CAD build for the part. Positions are in the model's coordinates, mm. A direction names the side the tool comes from. Give positions to 0.01 mm unless a question says otherwise; leave off trailing zeros. Order: outer loops, then holes, each group sorted by start corner. A loop starts at its lowest first (then second) coordinate and runs counter-clockwise, first axis right, second up. Notation, with made-up numbers: (24, 87.25) -> (83, 87.25) arc R25 cw to (83, 118.25) -> close; hole circle Ø9 at (1, 35). An arc over 180 degrees is marked (long way). Use one line per item in the form item = value. Start each with the question number.
1) Tool access for faces 4 (the face through (-4.705, -8, 7)), 5 (the face through (-22.305, 10, 7)), 6 (the face through (-1.188, -8, 7)): list every direction of +Z, -Z, +X, -X, +Y, -Y with a clear straight run to the whole face (end or side of a thin tool).
2) Cut at A-A, the plane x = -3.75. Give the cut face in (y, z).
3) Drop flat-ended pins along their axis: P1, Ø3, axis at y = -5, z = 4, coming from the +X side; P2, Ø4.5, axis at x = -10.5, z = 8.5, coming from the -Y side; P3, Ø4, axis at y = -9, z = 6, coming from the -X side; P4, Ø1.5, axis at x = -7, y = 5.5, coming from the -Z side. Give the stop position or say it passes through.
4) Cut at B-B, the plane y = 12. Give the cut face in (x, z).
5) Cut at C-C, the plane z = 1. Give the cut face in (x, y), and give its area (3 significant figures).
6) Probe line 1 (Y direction, x = -10.25, z = 9); line 2 (X direction, y = -4, z = 14); line 3 (X direction, y = 8, z = 13.5). List the from-to ranges inside material, lowest first.
7) Mould opens along X. For faces 1 (the face through (-24.007, -8, 7)), 2 (the face through (0.614, -0.124, 7.395)), 3 (the face through (-12, -0.694, 7)) say: pulls with the +X half, pulls with the -X half, needs draft (parallel to the pull), parting line crosses it, or undercut.
from build123d import *

# Parameters (mm, degrees)
SKETCH1_W           = 20
SKETCH1_H           = 13.5
BOSS_EXTRUDE1_DEPTH = 15
FILLET1_R           = 2


with BuildPart() as part:
    # Sketch1 → Boss-Extrude1 (new body)
    with BuildSketch(Plane.XY):
        Polygon((-25.825109991, 19.935146109), (1.215675598, 19.935146109), (1.215675598, -0.694178906), (-1.188139158, -0.694178906), (-1.188139158, -14.694178906), (-1.542833918, -14.694178906), (-4.704717196, -14.694178906), (-4.704717196, -0.694178906), (-19.904717196, -0.694178906), (-19.904717196, -14.694178906), (-24.006835368, -14.694178906), (-24.006835368, -0.694178906), (-25.825109991, -0.694178906), align=None)
        with Locations((-12.304717196, 9.620483601)):
            Rectangle(SKETCH1_W, SKETCH1_H, mode=Mode.SUBTRACT)
    extrude(amount=BOSS_EXTRUDE1_DEPTH)

    # Fillet1
    # the kernel refuses this fillet: 2 mm, written as the material it takes off along each edge
    with BuildSketch(Plane(origin=(-25.825109991, -0.694178906, -4.979317152), x_dir=(1, 0, 0), z_dir=(0, 0, 1))) as fillet1_piece_1:
        with BuildLine():
            CenterArc((2, 1.991726861), FILLET1_R, 180, 84.786761144)
            Line((0, 1.991726861), (-0.04, 1.991726861))
            Line((-0.04, 1.991726861), (-0.04, 0))
            Line((-0.04, 0), (0, -0.04))
            ThreePointArc((0, -0.04), (0.909137312, -0.04), (1.814640116, -0.039834537))
            Line((1.814640116, -0.039834537), (1.818274623, 0))
        make_face()
    extrude(amount=24.958634303, mode=Mode.SUBTRACT)
    with BuildSketch(Plane(origin=(-25.825109991, 19.935146109, -5), x_dir=(1, 0, 0), z_dir=(0, 0, 1)), Plane(origin=(1.215675598, -0.694178906, -5), x_dir=(-1, 0, 0), z_dir=(0, 0, 1))) as fillet1_piece_2:
        with BuildLine():
            CenterArc((FILLET1_R, -FILLET1_R), FILLET1_R, 90, 90)
            Line((0, -FILLET1_R), (-FILLET1_R * 0.02, -FILLET1_R))
            Line((-FILLET1_R * 0.02, -FILLET1_R), (-FILLET1_R * 0.02, FILLET1_R * 0.02))
            Line((-FILLET1_R * 0.02, FILLET1_R * 0.02), (FILLET1_R, FILLET1_R * 0.02))
            Line((FILLET1_R, FILLET1_R * 0.02), (FILLET1_R, 0))
        make_face()
    extrude(amount=25, mode=Mode.SUBTRACT)
    with BuildSketch(Plane(origin=(1.215675598, 19.935146109, -5), x_dir=(-1, 0, 0), z_dir=(0, 0, 1))) as fillet1_piece_3:
        with BuildLine():
            CenterArc((FILLET1_R, FILLET1_R), FILLET1_R, 180, 90)
            Line((0, FILLET1_R), (-FILLET1_R * 0.02, FILLET1_R))
            Line((-FILLET1_R * 0.02, FILLET1_R), (-FILLET1_R * 0.02, -FILLET1_R * 0.02))
            Line((-FILLET1_R * 0.02, -FILLET1_R * 0.02), (FILLET1_R, -FILLET1_R * 0.02))
            Line((FILLET1_R, -FILLET1_R * 0.02), (FILLET1_R, 0))
        make_face()
    extrude(amount=25, mode=Mode.SUBTRACT)


solid = part.part
Result:
q1.face_4 = +Z, -Z, -Y
q1.face_5 = +Z, -Z
q1.face_6 = +Z, -Z, +X, -Y
q2.outline = (-14.69, 0) -> (2.87, 0) -> (2.87, 15) -> (-14.69, 15) -> close; (16.37, 0) -> (19.94, 0) -> (19.94, 15) -> (16.37, 15) -> close
q3.P1 = -1.19
q3.P2 = -0.69
q3.P3 = -24.01
q3.P4 = through
q4.outline = (-25.83, 0) -> (-22.3, 0) -> (-22.3, 15) -> (-25.83, 15) -> close; (-2.3, 0) -> (1.22, 0) -> (1.22, 15) -> (-2.3, 15) -> close
q5.outline = (-25.83, 1.3) arc R2 ccw to (-24.01, -0.69) -> (-24.01, -14.69) -> (-19.9, -14.69) -> (-19.9, -0.69) -> (-4.7, -0.69) -> (-4.7, -14.69) -> (-1.19, -14.69) -> (-1.19, -0.69) -> (-0.78, -0.69) arc R2 ccw to (1.22, 1.31) -> (1.22, 17.94) arc R2 ccw to (-0.78, 19.94) -> (-23.83, 19.94) arc R2 ccw to (-25.83, 17.94) -> close; hole (-22.3, 2.87) -> (-2.3, 2.87) -> (-2.3, 16.37) -> (-22.3, 16.37) -> close
q5.area = 391 mm²
q6.line_1 = -0.69 to 2.87, 16.37 to 19.94
q6.line_2 = -24.01 to -19.9, -4.7 to -1.19
q6.line_3 = -25.83 to -22.3, -2.3 to 1.22
q7.face_1 = pulls with the -X half
q7.face_2 = pulls with the +X half
q7.face_3 = undercut
